from build123d import *

# Parameters (mm, degrees)
F0_W      = 59
F0_H      = 51.5
F1_DEPTH  = 26.8
F3_DEPTH  = 51.501
F4_W      = 13
F4_H      = 13
F5_DEPTH  = 22.75
F6_W      = 13
F6_H      = 3
F7_DEPTH  = 5
F9_W      = 10
F9_H      = 8.67
F10_DEPTH = 51.501


with BuildPart() as f1:
    # F0 (on Top) → F1 (new body)
    with BuildSketch(Plane.XY):
        Rectangle(F0_W, F0_H)
    extrude(amount=F1_DEPTH)

    # F2 (on face) → F3 (cut, through all)
    with BuildSketch(Plane.XZ.offset(25.75)):
        Polygon((10.242246, 26.8), (29.5, 0), (29.5, 26.8), align=None)
        Polygon((-29.5, 26.8), (-29.5, 0), (-10.242246, 26.8), align=None)
    extrude(amount=-F3_DEPTH, mode=Mode.SUBTRACT)

    # F4 (on face) → F5 (cut)
    with BuildSketch(Plane.XY.offset(26.8)):
        with Locations((0.104, -19.25)):
            Rectangle(F4_W, F4_H)
    extrude(amount=-F5_DEPTH, mode=Mode.SUBTRACT)

    # F6 (on face) → F7 (cut)
    with BuildSketch(Plane.XZ.offset(12.75)):
        with Locations((0.104, 23.3)):
            Rectangle(F6_W, F6_H)
    extrude(amount=-F7_DEPTH, mode=Mode.SUBTRACT)

    # F9 (on face) → F10 (cut, through all)
    with BuildSketch(Plane.XZ.offset(25.75)):
        with Locations((0.08, 4.335)):
            Rectangle(F9_W, F9_H)
    extrude(amount=-F10_DEPTH, mode=Mode.SUBTRACT)


solid = f1.part
Here's how the part is built. I have some questions about the finished solid (model axes, mm). A direction names the side the tool comes from. Give positions to 0.01 mm unless a question says otherwise; leave off trailing zeros. Order: outer loops, then holes, each group sorted by start corner. A loop starts at its lowest first (then second) coordinate and runs counter-clockwise, first axis right, second up. Notation, with made-up numbers: M 21.5,56.25 L 74.5,56.25 A27 ccw 74.5,74.25 Z; hole C -9,27.5 d10. An arc over 180 degrees is marked long. Answer as a JSON object with one key per item and string values. Group by question number.
1) We'd pull the mould along X, two halves only. Please class faces 5 (the flat face through (-6, -19, 4.05)), 6 (the flat face through (0, 25.75, 10)), 7 (the flat face through (-20.01, -0.36, 13.21)): pulls with the +X half, pulls with the -X half, needs draft (parallel to the pull), parting line crosses it, or undercut.
2) Suppose I cut it at B-B, the plane z = 3.25. Write out the boundary of the cut face in (x, y), plus the area to 3 significant figures.
3) Suppose I cut it at C-C, the plane y = -4.5. Write out the boundary of the cut face in (x, z).
4) I'm going to push flat-ended pins straight in: pin 1 Ø2 at (x, z) = (-1, 25.5) entering from -Y; pin 2 Ø5.5 at (y, z) = (-13.5, 18) entering from +X; pin 3 Ø2 at (x, y) = (-23.5, 3.5) entering from +Z. Where does each tip first touch, or does it pass through?
5) On a 3-axis mill with a long thin cutter (end or side, diameter ignored), from which of +Z, -Z, +X, -X, +Y, -Y can I reach the whole of each face in a straight line? I mean faces 1 (the flat face through (0, -12.75, 26)), 2 (the flat face through (-4.92, 0, 4)), 3 (the flat face through (0, -10, 21.8)), 4 (the flat face through (0, 0, 26.8)). Say none if no direction works.
6) Suppose I cut it at D-D, the plane z = 12. Write out the boundary of the cut face in (x, y).
7) Please list where these lines run through material, in increasing order: L1, parallel to X at y = -21, z = 12; L2, parallel to X at y = -20, z = 3; L3, parallel to Y at x = 0.5, z = 14.25. Write a range as [from, to].
8) Suppose I cut it at A-A, the plane y = -13.5. Write out the boundary of the cut face in (x, z), plus the area to 3 significant figures.
Results found:
{
 "1": {"face 5": "undercut", "face 6": "needs draft", "face 7": "pulls with the -X half"},
 "2": {"outline": "M -27.16,-25.75 L -4.92,-25.75 L -4.92,25.75 L -27.16,25.75 Z; M 5.08,-25.75 L 27.16,-25.75 L 27.16,25.75 L 5.08,25.75 Z", "area": "2,280 mm²"},
 "3": {"outline": "M -29.5,0 L -4.92,0 L -4.92,8.67 L 5.08,8.67 L 5.08,0 L 29.5,0 L 10.24,26.8 L -10.24,26.8 Z"},
 "4": {"pin 1": "y = -12.75", "pin 2": "x = 18.54", "pin 3": "z = 9.74"},
 "5": {"face 1": "+Z, -Y", "face 2": "-Z, +Y, -Y", "face 3": "-Y", "face 4": "+Z, +X, -X, +Y, -Y"},
 "6": {"outline": "M -20.88,-25.75 L -6.4,-25.75 L -6.4,-12.75 L 6.6,-12.75 L 6.6,-25.75 L 20.88,-25.75 L 20.88,25.75 L -20.88,25.75 Z"},
 "7": {"L1": "[-20.88, -6.4], [6.6, 20.88]", "L2": "[-27.34, -4.92], [5.08, 27.34]", "L3": "[-12.75, 25.75]"},
 "8": {"outline": "M -29.5,0 L -4.92,0 L -4.92,4.05 L -6.4,4.05 L -6.4,26.8 L -10.24,26.8 Z; M 5.08,0 L 29.5,0 L 10.24,26.8 L 6.6,26.8 L 6.6,4.05 L 5.08,4.05 Z", "area": "729 mm²"}
}
